Verification items for the finished model (mm, model axes). Face numbers are marked on the shaded views. A direction names the side the tool comes from. Round coordinates to 2 decimals unless told otherwise and drop trailing zeros. Loops run counter-clockwise (first coordinate to the right, second up) from the corner with the lowest first, then second, coordinate; pieces in that order, holes last.
from build123d import *

# Parameters (mm, degrees)
EXTRUDE_1_DEPTH = 2
SKETCH_2_W      = 0.5
SKETCH_2_H      = 20
SKETCH_2_W_2    = 10
SKETCH_2_H_2    = 0.5
EXTRUDE_2_DEPTH = 4
CHAMFER_1_SIZE  = 4
FILLET_1_R      = 2


with BuildPart() as part:
    # Эскиз1 → Бобышка-Вытянуть1 (new body)
    with BuildSketch(Plane.XY):
        with BuildLine():
            Line((-25.809245543, -34.533993398), (-22.574730597, -34.533993398))
            Line((-22.574730597, -34.533993398), (-19.086915297, -34.533993398))
            Line((-19.086915297, -34.533993398), (-15.809245543, -34.533993398))
            ThreePointArc((-15.809245543, -34.533993398), (-10.152391293, -32.190847647), (-7.809245543, -26.533993398))
            Line((-7.809245543, -26.533993398), (-7.809245543, -18.565345077))
            Line((-7.809245543, -18.565345077), (-7.809245543, -14.503170045))
            Line((-7.809245543, -14.503170045), (-7.809245543, -6.533993398))
            ThreePointArc((-7.809245543, -6.533993398), (-10.152391293, -0.877139148), (-15.809245543, 1.466006602))
            Line((-15.809245543, 1.466006602), (-19.086915297, 1.466006602))
            Line((-19.086915297, 1.466006602), (-22.574730597, 1.466006602))
            Line((-22.574730597, 1.466006602), (-25.809245543, 1.466006602))
            ThreePointArc((-25.809245543, 1.466006602), (-31.466099792, -0.877139148), (-33.809245543, -6.533993398))
            Line((-33.809245543, -6.533993398), (-33.809245543, -14.503170045))
            Line((-33.809245543, -14.503170045), (-33.809245543, -18.565345077))
            Line((-33.809245543, -18.565345077), (-33.809245543, -26.533993398))
            ThreePointArc((-33.809245543, -26.533993398), (-31.466099792, -32.190847647), (-25.809245543, -34.533993398))
        make_face()
    extrude(amount=EXTRUDE_1_DEPTH)

    # Эскиз2 → Бобышка-Вытянуть2 (add)
    with BuildSketch(Plane.XY.offset(2)):
        with Locations((-30.559245543, -16.533993398)):
            Rectangle(SKETCH_2_W, SKETCH_2_H)
        with Locations((-20.809245543, -31.283993398)):
            Rectangle(SKETCH_2_W_2, SKETCH_2_H_2)
        with Locations((-11.059245543, -16.533993398)):
            Rectangle(SKETCH_2_W, SKETCH_2_H)
        with Locations((-20.809245543, -1.783993398)):
            Rectangle(SKETCH_2_W_2, SKETCH_2_H_2)
    extrude(amount=EXTRUDE_2_DEPTH)

    # Фаска1
    chamfer_1_edges = [part.edges().sort_by_distance(p)[0] for p in [
        (-20.809245543, -31.033993398, 2),
        (-30.309245543, -16.533993398, 2),
        (-20.809245543, -2.033993398, 2),
        (-11.309245543, -16.533993398, 2),
    ]]
    chamfer(chamfer_1_edges, length=CHAMFER_1_SIZE - 0.0001)  # a hair under: the kernel refuses the full size

    # Скругление1
    fillet_1_edges = [part.edges().sort_by_distance(p)[0] for p in [
        (-31.466099792, -0.877139148, 0),
        (-20.809245543, 1.466006602, 0),
        (-10.152391293, -0.877139148, 0),
        (-7.809245543, -16.533993398, 0),
        (-10.152391293, -32.190847647, 0),
        (-20.809245543, -34.533993398, 0),
        (-31.466099792, -32.190847647, 0),
        (-33.809245543, -16.533993398, 0),
    ]]
    fillet(fillet_1_edges, radius=FILLET_1_R - 0.0001)  # a hair under: the kernel refuses the full size


solid = part.part
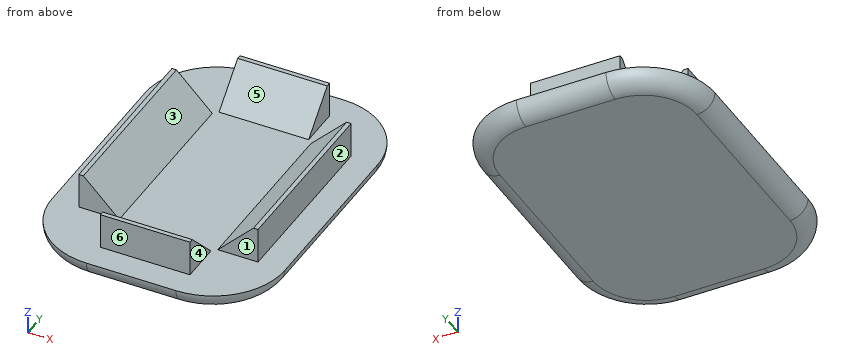
1. Scan lines: L1, parallel to Z at x = -25.75, y = -11.5; L2, parallel to X at y = -21.5, z = 2.5; L3, parallel to X at y = -22.5, z = 3.15. Record each from-to range of solid material in increasing order.
2. Section check A-A (z = 3.85). Enter the section's corners in (x, y), then the cut area to 3 significant figures.
3. Section check D-D (z = 1). Enter the section's corners in (x, y).
4. Gauge pin test, flat ends, axial feed: P1, Ø1.2, axis at x = -12, z = 4.5, coming from the -Y side; P2, Ø2, axis at y = -28.5, z = 5, coming from the -X side; P3, Ø3, axis at x = -22, z = 5, coming from the +Y side; P4, Ø2, axis at y = -19, z = 4, coming from the -X side. Record the tip position at first contact, or that the pin passes through.
5. Tool access check on the marked faces 4, 5 and 6. Record the directions out of +Z, -Z, +X, -X, +Y, -Y that give a thin tool (end or side, any length) a straight path to the whole face; none if there is none.
6. Release check for a two-part mould opening along X. For the marked faces 1, 2 and 3 record: released by +X, released by -X, zero draft, split by the parting line, or undercut.
Taken from the geometry:
1. L1: z = 0 to 2
1. L2: x = -30.81 to -26.81, -14.81 to -10.81
1. L3: x = -30.81 to -27.46, -14.16 to -10.81
2. outline: (-30.81, -26.53) - (-28.16, -26.53) - (-28.16, -6.53) - (-30.81, -6.53) - close; (-25.81, -31.53) - (-15.81, -31.53) - (-15.81, -28.88) - (-25.81, -28.88) - close; (-25.81, -4.18) - (-15.81, -4.18) - (-15.81, -1.53) - (-25.81, -1.53) - close; (-13.46, -26.53) - (-10.81, -26.53) - (-10.81, -6.53) - (-13.46, -6.53) - close
2. area: 159 mm2
3. outline: (-33.54, -26.53) arc R7.73 ccw to (-25.81, -34.27) - (-15.81, -34.27) arc R7.73 ccw to (-8.08, -26.53) - (-8.08, -6.53) arc R7.73 ccw to (-15.81, 1.2) - (-25.81, 1.2) arc R7.73 ccw to (-33.54, -6.53) - close
4. P1: stops at y = -26.53
4. P2: passes through
4. P3: stops at y = -1.53
4. P4: stops at x = -30.81
5. face 4: +Z, +X, +Y, -Y
5. face 5: +Z, +X, -X
5. face 6: +Z, +X, -X, -Y
6. face 1: zero draft
6. face 2: released by +X
6. face 3: undercut
